Geometry check sheet. Reference: drawing and pictorial views, mm from the part's lowest x, y, z. A direction names the side the tool comes from. Round coordinates to 2 decimals unless told otherwise and drop trailing zeros. Order: outer loops, then holes, each group sorted by start corner. A loop starts at its lowest first (then second) coordinate and runs counter-clockwise, first axis right, second up.
(1) Sectioned sample at A-A (y = 6). Record the boundary of the cut face in (x, z), plus the area to 4 significant figures.
(2) Sectioned sample at C-C (x = 42). Record the boundary of the cut face in (y, z).
(3) Set-up check for the marked faces 4, 5 and 6: record each of +Z, -Z, +X, -X, +Y, -Y from which the full face is reachable in a straight line by a thin tool's end or side.
(4) Go/stop test with flat-tipped pins: pin 1 (4 mm diameter, centred on x = 49, y = 40, fed in from -Z); pin 2 (2.5 mm diameter, centred on x = 58.5, z = 2.5, fed in from -Y); pin 3 (5.5 mm diameter, centred on x = 61, z = 3, fed in from +Y); pin 4 (1.5 mm diameter, centred on y = 21, z = 2.5, fed in from +X). Record where each tip stops, or that it passes through.
(5) Sectioned sample at B-B (z = 7.75). Record the boundary of the cut face in (x, y).
(6) Material ranges on line 1 along Y through (x, z) = (64, 8.25); line 2 along X through (y, z) = (33, 1.75); line 3 along Y through (x, z) = (52.5, 8.75), recorded low to high.
(7) Sectioned sample at D-D (x = 10.5). Record the boundary of the cut face in (y, z), plus the area to 3 significant figures.
(8) Release check for a two-part mould opening along X. For the marked faces 1, 2 and 3 record: +X half, -X half, draft (parallel to the pull), parting line (faces both ways), or undercut.
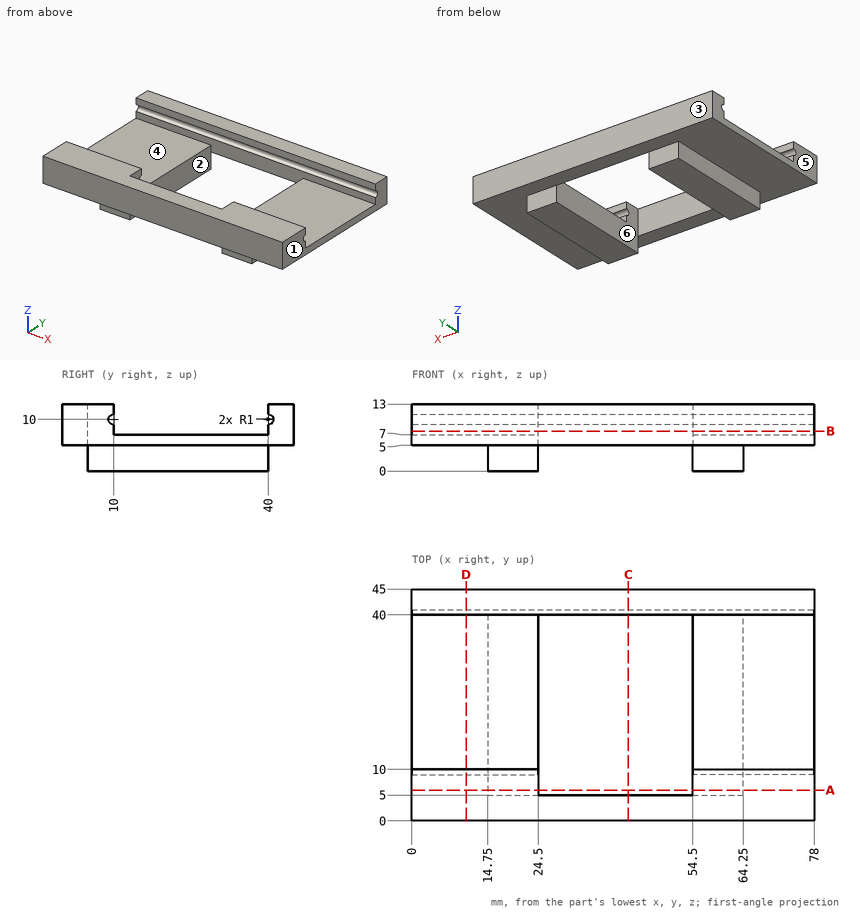
Answer below:
1. outline: (0, 5) - (14.75, 5) - (14.75, 0) - (24.5, 0) - (24.5, 13) - (0, 13) - close; (54.5, 0) - (64.25, 0) - (64.25, 5) - (78, 5) - (78, 13) - (54.5, 13) - close
1. area: 481.5 mm2
2. outline: (0, 5) - (5, 5) - (5, 13) - (0, 13) - close; (40, 5) - (45, 5) - (45, 13) - (40, 13) - (40, 11) arc R1 cw to (40, 9) - close
3. face 4: +Z, +X, -X
3. face 5: +Z, -Z, -X, +Y, -Y
3. face 6: +Z, -Z
4. pin 1: stops at z = 5
4. pin 2: stops at y = 5
4. pin 3: stops at y = 45
4. pin 4: stops at x = 64.25
5. outline: (0, 0) - (78, 0) - (78, 10) - (54.5, 10) - (54.5, 5) - (24.5, 5) - (24.5, 10) - (0, 10) - close; (0, 40) - (78, 40) - (78, 45) - (0, 45) - close
6. line 1: y = 0 to 10, 40 to 45
6. line 2: x = 14.75 to 24.5, 54.5 to 64.25
6. line 3: y = 0 to 5, 40 to 45
7. outline: (0, 5) - (45, 5) - (45, 13) - (40, 13) - (40, 11) arc R1 cw to (40, 9) - (40, 7) - (10, 7) - (10, 9) arc R1 cw to (10, 11) - (10, 13) - (0, 13) - close
7. area: 177 mm2
8. face 1: +X half
8. face 2: undercut
8. face 3: draft
